Here's how the part is built. I have some questions about the finished solid (model axes, mm). Round coordinates to 2 decimals unless told otherwise and drop trailing zeros. Write each loop counter-clockwise with the first axis right and the second up, starting at its lowest first coordinate (ties: lowest second). Pieces come first, ordered by that corner, then holes. Notation, with made-up numbers: (-16, 19.25) - (18, 19.25) arc R14 cw to (18, 40.25) - close; hole circle Ø3 at (22.5, 4). An arc over 180 degrees is marked (long way). Return JSON: item names as keys, results as strings. Group by question number.
Autodesk Inventor part; units mm, degrees
ref_plane "YZ Plane" through (0, 0, 0) normal (1, 0, 0) x (0, 1, 0)
ref_plane "XZ Plane" through (0, 0, 0) normal (0, 1, 0) x (-1, 0, 0)
ref_plane "XY Plane" through (0, 0, 0) normal (0, 0, 1) x (1, 0, 0)
sketch "Esboço1" plane through (0, 0, 0) normal (0, 0, 1) x (1, 0, 0)
  line L0 (-35, -75) -> (35, -75)
  line L1 (35, -75) -> (35, 75)
  line L2 (35, 75) -> (-35, 75)
  line L3 (-35, 75) -> (-35, -75)
  line L4 (-35, -75) -> (35, 75) construction
  line L5 (35, -75) -> (-35, 75) construction
  point P0 (0, 0)
  dimension "d0" = 150
  dimension "d1" = 70
extrude "Extrusão1" add sketch "Esboço1" along normal blind 4
sketch "Esboço2" plane through (0, 0, 4) normal (0, 0, 1) x (1, 0, 0)
  line L0 (35, 75) -> (-35, 75)
  line L1 (-35, -75) -> (35, -75)
  line L2 (-35, 75) -> (-35, -75)
  point P0 (0, 0)
  point P1 (0, 60)
  point P2 (0, -60)
  point P3 (0, 0)
  dimension "d4" = 15
  dimension "d5" = 15
  dimension "d6" = 35
  dimension "d7" = 35
hole "Furo1" at (0, 60, 4) at (0, -60, 4) at (0, 0, 4) direction (0, 0, -1) diameter 4.5 end through all countersink diameter 9.4 countersink angle 90
chamfer "Chanfro1" distance 2 angle 45 4 edges at (35, -75, 2) (-35, -75, 2) (35, 75, 2) (-35, 75, 2)
sketch "Esboço3" plane through (0, 0, 4) normal (0, 0, 1) x (1, 0, 0)
  circle A0 centre (34, -55) radius 1.5706
  circle A1 centre (34, -5) radius 1.5706
  circle A2 centre (-16, -55) radius 3.8 construction
  circle A3 centre (-16, -55) radius 2.2 construction
  circle A4 centre (-16, -5) radius 3.8 construction
  circle A5 centre (34, -55) radius 2.5
  circle A6 centre (34, -5) radius 2.5
  circle A7 centre (-16, -55) radius 2.5
  circle A8 centre (-16, -5) radius 2.5
  point P0 (0, 0)
  dimension "d18" = 5
extrude "Extrusão2" cut sketch "Esboço3" against normal blind 10 contours A0 | A1 | A5 | A6 | A7 | A8
fillet "Arredondamento1" radius 2 4 edges at (35, -2.7087, 2) (35, -7.2913, 2) (35, -52.7087, 2) (35, -57.2913, 2)
sketch "Esboço4" plane through (0, 0, 4) normal (0, 0, 1) x (1, 0, 0)
  circle A0 centre (9, -30) radius 5.5
  circle A1 centre (9, -30) radius 7.5
  point P0 (0, 0)
  dimension "d22" = 15
extrude "Extrusão3" cut sketch "Esboço4" against normal through all contours A0 | A1
properties part number "Espaçador módulo AC" material "Poliacetal"
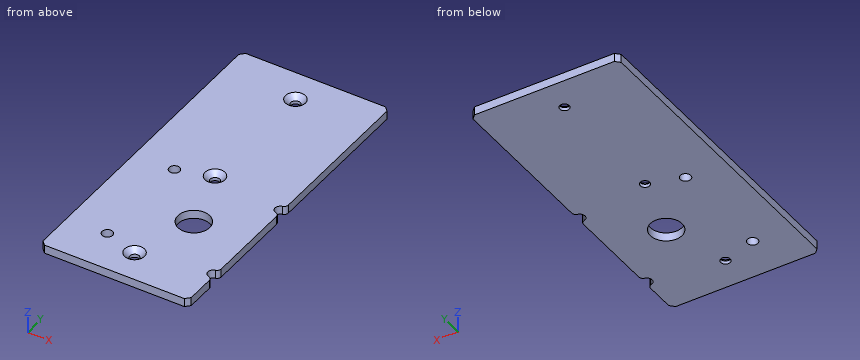
1) Will these pins go through, and if not, where does the flat tip stop? pin 1 Ø4.5 at (x, y) = (-16, -5) entering from -Z; pin 2 Ø7 at (x, y) = (0, 60) entering from +Z; pin 3 Ø8 at (x, y) = (-6.5, 40.5) entering from -Z; pin 4 Ø5 at (x, y) = (0, 0) entering from +Z.
2) Imagine slicing it at D-D (x = 0). Please give me the cut outline in (y, z), plus the area to 3 significant figures.
3) Imagine slicing it at C-C (z = 2.9). Please give me the cut outline in (x, y).
4) I need wall thicknesses on line 1 along Y through (x, z) = (-16.5, 0.35); line 2 along Y through (x, z) = (-16, 2.9); line 3 along Y through (x, z) = (0, 0.6). Which ranges of each line are inside material? Lowest first, please.
5) Imagine slicing it at A-A (x = -16). Please give me the cut outline in (y, z).
6) Imagine slicing it at B-B (y = 60). Please give me the cut outline in (x, z).
Results found:
{
 "1": {"pin 1": "passes through", "pin 2": "stops at z = 2.8", "pin 3": "stops at z = 0", "pin 4": "stops at z = 1.8"},
 "2": {"outline": "(-75, 0) - (-62.25, 0) - (-62.25, 1.55) - (-64.7, 4) - (-75, 4) - close; (-57.75, 0) - (-2.25, 0) - (-2.25, 1.55) - (-4.7, 4) - (-55.3, 4) - (-57.75, 1.55) - close; (2.25, 0) - (57.75, 0) - (57.75, 1.55) - (55.3, 4) - (4.7, 4) - (2.25, 1.55) - close; (62.25, 0) - (75, 0) - (75, 4) - (64.7, 4) - (62.25, 1.55) - close", "area": "528 mm²"},
 "3": {"outline": "(-35, -73) - (-33, -75) - (33, -75) - (35, -73) - (35, -59.39) arc R2 ccw to (33.44, -57.44) arc R2.5 cw to (33.44, -52.56) arc R2 ccw to (35, -50.61) - (35, -9.39) arc R2 ccw to (33.44, -7.44) arc R2.5 cw to (33.44, -2.56) arc R2 ccw to (35, -0.61) - (35, 73) - (33, 75) - (-33, 75) - (-35, 73) - close; hole circle Ø5 at (-16, -55); hole circle Ø5 at (-16, -5); hole circle Ø7.2 at (0, -60); hole circle Ø7.2 at (0, 0); hole circle Ø7.2 at (0, 60); hole circle Ø15 at (9, -30)"},
 "4": {"line 1": "y = -75 to -57.45, -52.55 to -7.45, -2.55 to 75", "line 2": "y = -75 to -57.5, -52.5 to -7.5, -2.5 to 75", "line 3": "y = -75 to -62.25, -57.75 to -2.25, 2.25 to 57.75, 62.25 to 75"},
 "5": {"outline": "(-75, 0) - (-57.5, 0) - (-57.5, 4) - (-75, 4) - close; (-52.5, 0) - (-7.5, 0) - (-7.5, 4) - (-52.5, 4) - close; (-2.5, 0) - (75, 0) - (75, 4) - (-2.5, 4) - close"},
 "6": {"outline": "(-35, 0) - (-2.25, 0) - (-2.25, 1.55) - (-4.7, 4) - (-35, 4) - close; (2.25, 0) - (35, 0) - (35, 4) - (4.7, 4) - (2.25, 1.55) - close"}
}
